Part model, mm, in its own coordinate system. Face numbers are marked on the shaded views. A direction names the side the tool comes from. Coordinates: 2 decimals unless noted, no trailing zeros. Loops run counter-clockwise (first coordinate to the right, second up) from the corner with the lowest first, then second, coordinate; pieces in that order, holes last. Notation, with made-up numbers: (43, 45) - (69, 45) arc R18 ccw to (69, 80) - close; hole circle Ø11 at (-4.5, 1). An arc over 180 degrees is marked (long way). Use a Markdown table: item, result. Add a question column.
1) Pull direction X, two halves, no side cores. Call the marked faces 1, 2 and 3: +X half, -X half, draft (parallel to the pull), parting line (faces both ways), or undercut.
2) Drop flat-ended pins along their axis: P1, Ø3, axis at y = 3.5, z = -11, coming from the +X side; P2, Ø3.5, axis at x = 3.5, z = -9, coming from the -Y side; P3, Ø2, axis at y = -4, z = -15, coming from the -X side; P4, Ø6, axis at x = 14.5, z = -17, coming from the +Y side. Give the stop position or say it passes through.
3) Tool access for the marked faces 4, 5, 6, 7 and 8: list every direction of +Z, -Z, +X, -X, +Y, -Y with a clear straight run to the whole face (end or side of a thin tool).
4) Band-saw the part on A-A (z = -9.25). Give the cut face in (x, y).
5) Band-saw the part on D-D (x = 6). Give the cut face in (y, z) (3 decimals), plus the area to 3 significant figures.
6) Band-saw the part on B-B (y = 10). Give the cut face in (x, z) (3 decimals), plus the area to 3 significant figures.
7) Band-saw the part on C-C (z = -5.5). Give the cut face in (x, y) (3 decimals), plus the area to 3 significant figures.
8) Probe probe 1 along X at (y, z) = (10, -3.8) (3 decimals); probe 2 along Z at (x, y) = (-8, 9); probe 3 along X at (y, z) = (10, -7.05) (3 decimals). List the from-to ranges inside material, lowest first. Write a range as [from, to].
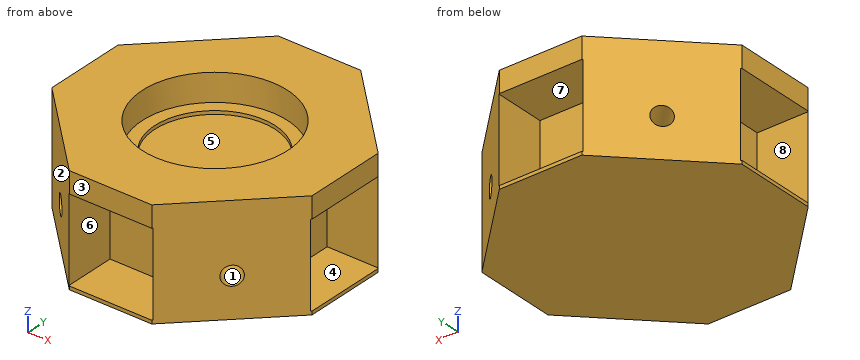
from build123d import *

# Parameters (mm, degrees)
SKIZZE1_W                          = 37.873435046
SKIZZE1_H                          = 37.873435047
AUFSATZ_LINEAR_AUSTRAGEN1_DEPTH    = 20
SKIZZE2_R                          = 10.575
SCHNITT_LINEAR_AUSTRAGEN1_DEPTH    = 4
SKIZZE3_W                          = 12
SKIZZE3_H                          = 12
SCHNITT_LINEAR_AUSTRAGEN3_DEPTH    = 7.5
VERRUNDUNG1_R                      = 8
KREISMUSTER1_COUNT                 = 4
SKIZZE4_R                          = 8.775
SCHNITT_LINEAR_AUSTRAGEN4_DEPTH    = 0.5
K_RPER_VERSCHIEBEN_KOPIEREN1_ANGLE = 90
SCHNITT_LINEAR_AUSTRAGEN5_DEPTH    = 44.118134258
SCHNITT_LINEAR_START               = -6
SKIZZE6_R                          = 1.4
SCHNITT_LINEAR_AUSTRAGEN6_DEPTH    = 16
KREISMUSTER2_COUNT                 = 4
SKIZZE7_W                          = 35.652729611
SKIZZE7_H                          = 9.373531579
SCHNITT_LINEAR_AUSTRAGEN8_DEPTH    = 51.066462265
SKIZZE8_W                          = 12.2
SKIZZE8_H                          = 12.2
SCHNITT_LINEAR_AUSTRAGEN9_DEPTH    = 7.5
KREISMUSTER11_COUNT                = 4


with BuildPart() as part:
    # Skizze1 → Aufsatz-Linear austragen1 (new body)
    with BuildSketch(Plane(origin=(0, 0, 0), x_dir=(1, 0, 0), z_dir=(0, 1, 0))):
        with Locations((6, 12.936717524)):
            Rectangle(SKIZZE1_W, SKIZZE1_H)
    extrude(amount=AUFSATZ_LINEAR_AUSTRAGEN1_DEPTH)

    # Skizze2 → Schnitt-Linear austragen1 (cut)
    with BuildSketch(Plane.XZ):
        with Locations(Location((6, -12.936717523, 0), (0, 0, 270))):
            Circle(SKIZZE2_R)
    extrude(amount=-SCHNITT_LINEAR_AUSTRAGEN1_DEPTH, mode=Mode.SUBTRACT)

    # Skizze3 → Schnitt-Linear austragen3 (cut)
    with BuildSketch(Plane.XY.offset(6)):
        with Locations((6, 9.2)):
            Rectangle(SKIZZE3_W, SKIZZE3_H)
    schnitt_linear_austragen3 = extrude(amount=-SCHNITT_LINEAR_AUSTRAGEN3_DEPTH, mode=Mode.SUBTRACT)

    # Verrundung1
    verrundung1_edges = [part.edges().sort_by_distance(p)[0] for p in [
        (24.936717523, 10, -31.873435047),
        (24.936717523, 10, 6),
        (-12.936717523, 10, 6),
        (-12.936717523, 10, -31.873435047),
    ]]
    fillet(verrundung1_edges, radius=VERRUNDUNG1_R)

    # Kreismuster1: Schnitt-Linear austragen3 ×4 about axis
    kreismuster1_axis = Axis((6, 0, -12.936717523), (0, 1, 0))
    for i in range(1, KREISMUSTER1_COUNT):
        add(schnitt_linear_austragen3.rotate(kreismuster1_axis, i * 360 / KREISMUSTER1_COUNT), mode=Mode.SUBTRACT)

    # Skizze4 → Schnitt-Linear austragen4 (cut)
    with BuildSketch(Plane.XZ.offset(-4)):
        with Locations(Location((6, -12.936717523, 0), (0, 0, 270))):
            Circle(SKIZZE4_R)
    extrude(amount=-SCHNITT_LINEAR_AUSTRAGEN4_DEPTH, mode=Mode.SUBTRACT)


with BuildPart() as part_1:
    # Körper-Verschieben/Kopieren1: moved
    add(part.part.rotate(Axis((0, 10, -12.936717523), (-1, 0, 0)), K_RPER_VERSCHIEBEN_KOPIEREN1_ANGLE))

    # Skizze5 → Schnitt-Linear austragen5 (cut, through all)
    with BuildSketch(Plane.XY.offset(-2.936717523)):
        Polygon((0, 28.936717523), (-12.936717523, 16), (-12.936717523, 28.936717523), align=None)
        Polygon((24.936717523, 16), (24.936717523, 28.936717523), (12, 28.936717523), align=None)
        Polygon((12, -8.936717523), (24.936717523, 4), (24.936717523, -8.936717523), align=None)
        Polygon((-12.936717523, -8.936717523), (0, -8.936717523), (-12.936717523, 4), align=None)
    extrude(amount=-SCHNITT_LINEAR_AUSTRAGEN5_DEPTH, mode=Mode.SUBTRACT)

    # Skizze6 → Schnitt-Linear austragen6 (cut)
    with BuildSketch(Plane(origin=(-14.468358762, 14.468358762, 0), x_dir=(0.7071067811865559, 0.7071067811865392, 0), z_dir=(-0.7071067811865392, 0.7071067811865559, 0)).offset(SCHNITT_LINEAR_START)):
        with Locations((11.284238529, 12.936717523)):
            Circle(SKIZZE6_R)
    schnitt_linear_austragen6 = extrude(amount=SCHNITT_LINEAR_AUSTRAGEN6_DEPTH, mode=Mode.SUBTRACT)

    # Kreismuster2: Schnitt-Linear austragen6 ×4 about axis
    kreismuster2_axis = Axis((6, 10, 0), (0, 0, 1))
    for i in range(1, KREISMUSTER2_COUNT):
        add(schnitt_linear_austragen6.rotate(kreismuster2_axis, i * 360 / KREISMUSTER2_COUNT), mode=Mode.SUBTRACT)

    # Skizze7 → Schnitt-Linear austragen8 (cut, through all)
    with BuildSketch(Plane(origin=(20.468358762, 20.468358762, 0), x_dir=(0.7071067811865558, -0.7071067811865392, 0), z_dir=(0.7071067811865392, 0.7071067811865558, 0))):
        with Locations((-3.021869868, 23.423483313)):
            Rectangle(SKIZZE7_W, SKIZZE7_H)
    extrude(amount=-SCHNITT_LINEAR_AUSTRAGEN8_DEPTH, mode=Mode.SUBTRACT)

    # Skizze8 → Schnitt-Linear austragen9 (cut)
    with BuildSketch(Plane.ZY.offset(12.936717523)):
        with Locations((-12.136717523, 10)):
            Rectangle(SKIZZE8_W, SKIZZE8_H)
    schnitt_linear_austragen9 = extrude(amount=-SCHNITT_LINEAR_AUSTRAGEN9_DEPTH, mode=Mode.SUBTRACT)

    # Kreismuster11: Schnitt-Linear austragen9 ×4 about axis
    kreismuster11_axis = Axis((6, 10, 0), (0, 0, 1))
    for i in range(1, KREISMUSTER11_COUNT):
        add(schnitt_linear_austragen9.rotate(kreismuster11_axis, i * 360 / KREISMUSTER11_COUNT), mode=Mode.SUBTRACT)


solid = part_1.part
Answer block:
| question | item | result |
|---|---|---|
| 1 | face 1 | undercut |
| 1 | face 2 | -X half |
| 1 | face 3 | draft |
| 2 | P1 | x = 24.84 |
| 2 | P2 | y = -1.44 |
| 2 | P3 | x = -5.94 |
| 2 | P4 | y = 28.94 |
| 3 | face 4 | +X |
| 3 | face 5 | +Z |
| 3 | face 6 | -Y |
| 3 | face 7 | +Y |
| 3 | face 8 | -X |
| 4 | outline | (-12.84, 3.9) - (-0.1, -8.84) - (-0.1, -1.44) - (12.1, -1.44) - (12.1, -8.84) - (24.84, 3.9) - (17.44, 3.9) - (17.44, 16.1) - (24.84, 16.1) - (12.1, 28.84) - (12.1, 21.44) - (-0.1, 21.44) - (-0.1, 28.84) - (-12.84, 16.1) - (-5.44, 16.1) - (-5.44, 3.9) - close |
| 5 | outline | (-8.937, -18.737) - (28.937, -18.737) - (28.937, -18.237) - (21.437, -18.237) - (21.437, -6.037) - (28.937, -6.037) - (28.937, -2.937) - (20.575, -2.937) - (20.575, -6.937) - (18.775, -6.937) - (18.775, -7.437) - (1.225, -7.437) - (1.225, -6.937) - (-0.575, -6.937) - (-0.575, -2.937) - (-8.937, -2.937) - (-8.937, -6.037) - (-1.437, -6.037) - (-1.437, -18.237) - (-8.937, -18.237) - close |
| 5 | area | 322 mm2 |
| 6 | outline | (-12.937, -18.737) - (24.937, -18.737) - (24.937, -18.237) - (17.437, -18.237) - (17.437, -6.037) - (24.937, -6.037) - (24.937, -2.937) - (16.575, -2.937) - (16.575, -6.937) - (14.775, -6.937) - (14.775, -7.437) - (-2.775, -7.437) - (-2.775, -6.937) - (-4.575, -6.937) - (-4.575, -2.937) - (-12.937, -2.937) - (-12.937, -6.037) - (-5.437, -6.037) - (-5.437, -18.237) - (-12.937, -18.237) - close |
| 6 | area | 322 mm2 |
| 7 | outline | (-12.937, 4) - (0, -8.937) - (12, -8.937) - (24.937, 4) - (24.937, 16) - (12, 28.937) - (0, 28.937) - (-12.937, 16) - close; hole circle Ø21.15 at (6, 10) |
| 7 | area | 748 mm2 |
| 8 | probe 1 | [-12.937, -4.575], [16.575, 24.937] |
| 8 | probe 2 | [-18.74, -18.24], [-6.04, -2.94] |
| 8 | probe 3 | [-5.437, -2.775], [14.775, 17.437] |
